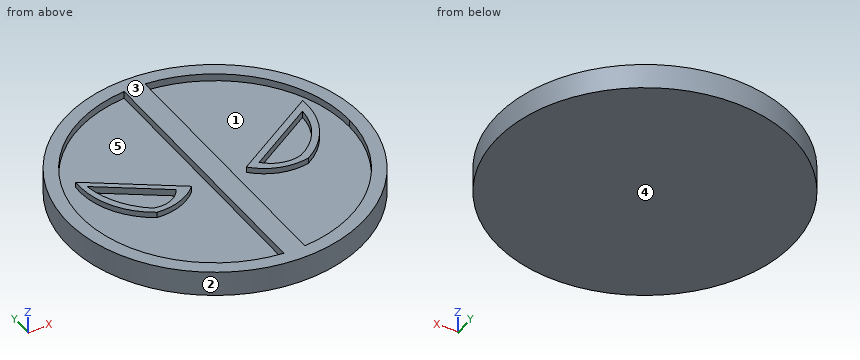
```python
from build123d import *

# Parameters (mm, degrees)
F0_R     = 72.129712
F1_DEPTH = 12.192
F2_DEPTH = 8.636
F3_DEPTH = 11.43
F4_DEPTH = 8.128


with BuildPart() as f1:
    # F0 (on Top) → F1 (new body)
    with BuildSketch(Plane.XY):
        Circle(F0_R)
        with BuildLine():
            ThreePointArc((4.806476, 65.403976), (48.04161, 44.640631), (65.580349, 0))
            ThreePointArc((65.580349, 0), (48.04161, -44.640631), (4.806476, -65.403976))
            ThreePointArc((4.806476, -65.403976), (-0.298713, -65.579669), (-5.40209, -65.357476))
            ThreePointArc((-5.40209, -65.357476), (-65.580349, 0), (-5.40209, 65.357476))
            ThreePointArc((-5.40209, 65.357476), (-0.298713, 65.579669), (4.806476, 65.403976))
        make_face(mode=Mode.SUBTRACT)
        with BuildLine():
            Line((4.806476, -65.403976), (4.806476, 65.403976))
            ThreePointArc((4.806476, 65.403976), (-0.298713, 65.579669), (-5.40209, 65.357476))
            Line((-5.40209, 65.357476), (-5.40209, -65.357476))
            ThreePointArc((-5.40209, -65.357476), (-0.298713, -65.579669), (4.806476, -65.403976))
        make_face()
    extrude(amount=F1_DEPTH)

    # F0 (on Top) → F2 (join)
    with BuildSketch(Plane.XY):
        with BuildLine():
            Line((-5.40209, -65.357476), (-5.40209, 65.357476))
            ThreePointArc((-5.40209, 65.357476), (-65.580349, 0), (-5.40209, -65.357476))
        make_face()
        with BuildLine():
            ThreePointArc((-35.997212, -12.835954), (-50.439117, 2.12982), (-54.568859, 22.513349))
            Line((-54.568859, 22.513349), (-14.25985, -4.810002))
            ThreePointArc((-14.25985, -4.810002), (-24.227117, -11.264353), (-35.997212, -12.835954))
        make_face(mode=Mode.SUBTRACT)
        with BuildLine():
            ThreePointArc((4.806476, -65.403976), (48.04161, -44.640631), (65.580349, 0))
            ThreePointArc((65.580349, 0), (48.04161, 44.640631), (4.806476, 65.403976))
            Line((4.806476, 65.403976), (4.806476, -65.403976))
        make_face()
        with BuildLine():
            ThreePointArc((37.965938, -12.946998), (24.058988, -12.403736), (12.256999, -5.027325))
            Line((12.256999, -5.027325), (56.192723, 22.513349))
            ThreePointArc((56.192723, 22.513349), (52.24232, 2.129374), (37.965938, -12.946998))
        make_face(mode=Mode.SUBTRACT)
    extrude(amount=F2_DEPTH)

    # F0 (on Top) → F3 (join)
    with BuildSketch(Plane.XY):
        with BuildLine():
            Line((-14.25985, -4.810002), (-54.568859, 22.513349))
            ThreePointArc((-54.568859, 22.513349), (-50.439117, 2.12982), (-35.997212, -12.835954))
            ThreePointArc((-35.997212, -12.835954), (-24.227117, -11.264353), (-14.25985, -4.810002))
        make_face()
        with BuildLine():
            ThreePointArc((-35.997212, -9.472951), (-46.80737, 2.354515), (-51.982607, 17.519125))
            Line((-51.982607, 17.519125), (-21.073241, -3.432703))
            ThreePointArc((-21.073241, -3.432703), (-27.461786, -9.105034), (-35.997212, -9.472951))
        make_face(mode=Mode.SUBTRACT)
        with BuildLine():
            Line((56.192723, 22.513349), (12.256999, -5.027325))
            ThreePointArc((12.256999, -5.027325), (24.058988, -12.403736), (37.965938, -12.946998))
            ThreePointArc((37.965938, -12.946998), (52.24232, 2.129374), (56.192723, 22.513349))
        make_face()
        with BuildLine():
            Line((18.524186, -5.007584), (52.319836, 16.176885))
            ThreePointArc((52.319836, 16.176885), (47.754564, 0.943554), (35.997216, -9.764426))
            ThreePointArc((35.997216, -9.764426), (26.574656, -9.906012), (18.524186, -5.007584))
        make_face(mode=Mode.SUBTRACT)
    extrude(amount=F3_DEPTH)

    # F0 (on Top) → F4 (join)
    with BuildSketch(Plane.XY):
        with BuildLine():
            Line((-21.073241, -3.432703), (-51.982607, 17.519125))
            ThreePointArc((-51.982607, 17.519125), (-46.80737, 2.354515), (-35.997212, -9.472951))
            ThreePointArc((-35.997212, -9.472951), (-27.461786, -9.105034), (-21.073241, -3.432703))
        make_face()
        with BuildLine():
            ThreePointArc((35.997216, -9.764426), (47.754564, 0.943554), (52.319836, 16.176885))
            Line((52.319836, 16.176885), (18.524186, -5.007584))
            ThreePointArc((18.524186, -5.007584), (26.574656, -9.906012), (35.997216, -9.764426))
        make_face()
    extrude(amount=F4_DEPTH)


solid = f1.part
```
Input: part model. Units: mm. Frame: model coordinates. Face numbers are marked on the shaded views. A direction names the side the tool comes from. Coordinates: 2 decimals unless noted, no trailing zeros. Loops run counter-clockwise (first coordinate to the right, second up) from the corner with the lowest first, then second, coordinate; pieces in that order, holes last. Notation, with made-up numbers: (-5.5, 37) -> (37.5, 37) arc R21 cw to (37.5, 46) -> close; hole circle Ø8 at (24, -31.75). An arc over 180 degrees is marked (long way). Use a Markdown table: item, result.
1) Contact query for flat-ended pins moving along their axis: pin 1 (6 mm diameter, centred on x = -36.5, z = 4.5, fed in from -Y); pin 2 (1 mm diameter, centred on y = -30, z = 10.5, fed in from -X); pin 3 (5 mm diameter, centred on y = -52, z = 9, fed in from -X). Output: stop coordinate, or through.
Results found:
| item | result |
|---|---|
| pin 1 | stops at y = -63.88 |
| pin 2 | stops at x = -65.82 |
| pin 3 | stops at x = -52.46 |
2) Cut plane A-A (y = -30). Return the cut outline in (x, z), then the cut area to 3 significant figures.
Results found:
| item | result |
|---|---|
| outline | (-65.59, 0) -> (65.59, 0) -> (65.59, 12.19) -> (58.32, 12.19) -> (58.32, 8.64) -> (4.81, 8.64) -> (4.81, 12.19) -> (-5.4, 12.19) -> (-5.4, 8.64) -> (-58.32, 8.64) -> (-58.32, 12.19) -> (-65.59, 12.19) -> close |
| area | 1,220 mm2 |
3) Cut plane C-C (x = 49.5). Return the cut outline in (y, z), then the cut area to 3 significant figures.
Results found:
| item | result |
|---|---|
| outline | (-52.46, 0) -> (52.46, 0) -> (52.46, 12.19) -> (43.02, 12.19) -> (43.02, 8.64) -> (18.32, 8.64) -> (18.32, 11.43) -> (14.41, 11.43) -> (14.41, 8.13) -> (4.13, 8.13) -> (4.13, 11.43) -> (-2.38, 11.43) -> (-2.38, 8.64) -> (-43.02, 8.64) -> (-43.02, 12.19) -> (-52.46, 12.19) -> close |
| area | 997 mm2 |
4) Access query for the marked faces 4 and 5. Directions: +Z, -Z, +X, -X, +Y, -Y. A direction counts if a zero-diameter tool reaches every point of the face in a straight line with its end or side. Return the directions, or none.
Results found:
| item | result |
|---|---|
| face 4 | -Z, +X, -X, +Y, -Y |
| face 5 | +Z |
5) Material intervals for line 1 along X through (y, z) = (32.5, 10); line 2 along Y through (x, z) = (-27, 10); line 3 along Z through (x, y) = (8, -55), sorted ascending. Write a range as from..to.
Results found:
| item | result |
|---|---|
| line 1 | x = -64.39..-56.96, -5.4..4.81, 56.96..64.39 |
| line 2 | y = -66.89..-59.76, -12.12..-8.91, 0.58..3.83, 59.76..66.89 |
| line 3 | z = 0..8.64 |
6) Pull-direction query (X, two-part tool) for the marked faces 1, 2 and 3; classes: released by +X, released by -X, zero draft, split by the parting line, or undercut.
Results found:
| item | result |
|---|---|
| face 1 | undercut |
| face 2 | split by the parting line |
| face 3 | zero draft |
7) Cut plane B-B (x = 14.5). Return the cut outline in (y, z).
Results found:
| item | result |
|---|---|
| outline | (-70.66, 0) -> (70.66, 0) -> (70.66, 12.19) -> (63.96, 12.19) -> (63.96, 8.64) -> (-3.62, 8.64) -> (-3.62, 11.43) -> (-7.16, 11.43) -> (-7.16, 8.64) -> (-63.96, 8.64) -> (-63.96, 12.19) -> (-70.66, 12.19) -> close |
